```python
from build123d import *

# Parameters (mm, degrees)
SKETCH2_R           = 15
BOSS_EXTRUDE1_DEPTH = 360


with BuildPart() as part:
    # Sketch1 → Revolve1 (revolve)
    with BuildSketch(Plane.XY, mode=Mode.PRIVATE) as revolve1_sk:
        Polygon((-855, 0), (-855, 215), (-830, 215), (-830, 240), (-730, 240), (-705, 160), (-705, 90), (-606.156213382, 90), (-606.156213382, 75), (-129.903810568, 75), (129.903810568, 75), (606.156213382, 75), (606.156213382, 90), (705, 90), (705, 160), (730, 240), (830, 240), (830, 215), (855, 215), (855, 0), align=None)
    revolve(revolve1_sk.sketch.rotate(Axis((-1250, 0, 0), (1, 0, 0)), 90), axis=Axis((-1250, 0, 0), (1, 0, 0)))

    # Sketch2 → Boss-Extrude1 (add)
    with BuildSketch(Plane.ZY.offset(855)):
        with Locations(Location((0, 150, 0), (0, 0, 180))):
            Circle(SKETCH2_R)
        with Locations(Location((106.066017178, 106.066017178, 0), (0, 0, 180))):
            Circle(SKETCH2_R)
        with Locations(Location((150, 0, 0), (0, 0, 180))):
            Circle(SKETCH2_R)
        with Locations(Location((106.066017178, -106.066017178, 0), (0, 0, 180))):
            Circle(SKETCH2_R)
        with Locations(Location((0, -150, 0), (0, 0, 180))):
            Circle(SKETCH2_R)
        with Locations(Location((-106.066017178, -106.066017178, 0), (0, 0, 180))):
            Circle(SKETCH2_R)
        with Locations(Location((-150, 0, 0), (0, 0, 180))):
            Circle(SKETCH2_R)
        with Locations(Location((-106.066017178, 106.066017178, 0), (0, 0, 180))):
            Circle(SKETCH2_R)
    boss_extrude1 = extrude(amount=BOSS_EXTRUDE1_DEPTH)

    # Mirror1: Boss-Extrude1 across plane
    add(boss_extrude1.mirror(Plane(origin=(0, 0, 0), x_dir=(0, 0, 1), z_dir=(1, 0, 0))))


solid = part.part
```
Verification items for the finished model (mm, model axes). A direction names the side the tool comes from. Give positions to 0.01 mm unless a question says otherwise; leave off trailing zeros. Order: outer loops, then holes, each group sorted by start corner. A loop starts at its lowest first (then second) coordinate and runs counter-clockwise, first axis right, second up. Notation, with made-up numbers: M 5,-19 L 44,-19 A20 cw 44,3 Z; hole C 65.25,-15.75 d11. An arc over 180 degrees is marked long. Answer in a Markdown table with one row per item. Add a question column.
Item 1: Scan lines: probe 1 along X at (y, z) = (85.5, -81); probe 2 along X at (y, z) = (79, -28.5); probe 3 along Z at (x, y) = (-80, 35). Record each from-to range of solid material in increasing order. Write a range as from..to.
Item 2: Mould release check, pull along X, two halves, no side actions. Record for faces 1 (the flat face through (830, -90, -197)), 2 (the cylindrical face through (-779.3, -202.37, 129.02)), 3 (the conical face through (706.564, -49.563, 157.385)), 4 (the flat face through (-855, -3, 3)): released by +X, released by -X, zero draft, split by the parting line, or undercut.
Item 3: Section check A-A, the plane x = 149. Enter the section's corners in (y, z), and give its area (3 significant figures).
Item 4: Gauge pin test, flat ends, axial feed: pin 1 (1 mm diameter, centred on y = 89.5, z = -56, fed in from +X); pin 2 (2 mm diameter, centred on x = -796.5, z = 111.5, fed in from -Y); pin 3 (10 mm diameter, centred on x = -122.5, z = -43.5, fed in from -Y). Record the tip position at first contact, or that the pin passes through.
Item 5: Tool access check on faces 5 (the cylindrical face through (780.7, -202.37, 129.02)), 6 (the flat face through (-830, -90, 197)), 7 (the flat face through (-705, 69, 69)), 8 (the flat face through (855, -3, -3)). Record the directions out of +Z, -Z, +X, -X, +Y, -Y that give a thin tool (end or side, any length) a straight path to the whole face; none if there is none.
Filled sheet:
| question | item | result |
|---|---|---|
| 1 | probe 1 | x = -855..-705, 705..855 |
| 1 | probe 2 | x = -855..-606.16, 606.16..855 |
| 1 | probe 3 | z = -66.33..66.33 |
| 2 | face 1 | released by +X |
| 2 | face 2 | zero draft |
| 2 | face 3 | undercut |
| 2 | face 4 | released by -X |
| 3 | outline | C 0,0 d150 |
| 3 | area | 17,700 mm^2 |
| 4 | pin 1 | stops at x = 855 |
| 4 | pin 2 | stops at y = -213.05 |
| 4 | pin 3 | stops at y = -64.36 |
| 5 | face 5 | +X, -X |
| 5 | face 6 | -X |
| 5 | face 7 | none |
| 5 | face 8 | +X |
